Autodesk Inventor part; units mm, degrees
ref_plane "YZ Plane" through (0, 0, 0) normal (1, 0, 0) x (0, 1, 0)
ref_plane "XZ Plane" through (0, 0, 0) normal (0, 1, 0) x (-1, 0, 0)
ref_plane "XY Plane" through (0, 0, 0) normal (0, 0, 1) x (1, 0, 0)
sketch "Эскиз1" plane through (0, 0, 0) normal (1, 0, 0) x (0, 1, 0)
  line L0 (70.9825, 98.2222) -> (-59.0175, 98.2222)
  line L1 (-59.0175, 98.2222) -> (-59.0175, -105.7778)
  line L2 (-59.0175, -105.7778) -> (70.9825, -105.7778)
  line L3 (70.9825, -105.7778) -> (70.9825, 98.2222)
  circle A0 centre (-34.0175, 95.2222) radius 1.5
  circle A1 centre (-34.0175, -102.7778) radius 1.5
  circle A2 centre (12.9825, 95.2222) radius 1.5
  circle A3 centre (12.9825, -102.7778) radius 1.5
  circle A4 centre (32.9825, 95.2222) radius 1.5
  circle A5 centre (32.9825, -102.7778) radius 1.5
  line L4 (-59.0175, -105.7778) -> (70.9825, -105.7778)
  line L5 (70.9825, -105.7778) -> (70.9825, -127.7504)
  line L6 (70.9825, -127.7504) -> (-59.0175, -127.7504)
  line L7 (-59.0175, -127.7504) -> (-59.0175, -105.7778)
  point P0 (0, 0)
  dimension "d0" = 204
  dimension "d1" = 130
  dimension "d2" = 3
  dimension "d3" = 25
  dimension "d4" = 25
  dimension "d5" = 3
  dimension "d6" = 3
  dimension "d7" = 3
  dimension "d8" = 72
  dimension "d9" = 3
  dimension "d10" = 3
  dimension "d11" = 3
  dimension "d12" = 72
  dimension "d13" = 3
  dimension "d14" = 3
  dimension "d15" = 20
  dimension "d16" = 3
  dimension "d17" = 3
  dimension "d18" = 20
extrude "Выдавливание1" add sketch "Эскиз1" along normal blind 4
sketch "Эскиз2" plane through (0, 0, 0) normal (-1, 0, 0) x (0, 0, 1)
  circle A0 centre (-112.7504, -20.3037) radius 1.5
  circle A1 centre (25.0776, -20.3037) radius 1.5
  line L0 (98.2222, -59.0175) -> (-105.7778, -59.0175)
  circle A2 centre (-112.7504, 39.6963) radius 1.5
  circle A3 centre (25.0776, 39.6963) radius 1.5
  line L1 (98.2222, 70.9825) -> (98.2222, -59.0175)
  circle A4 centre (-102.7778, 12.9825) radius 1.5
  line L2 (-105.7778, -59.0175) -> (-105.7778, 70.9825)
  line L3 (-105.7778, 70.9825) -> (98.2222, 70.9825)
  line L4 (-127.7504, -59.0175) -> (-127.7504, 70.9825)
  circle A5 centre (-30.9224, 29.6963) radius 1.5
  point P0 (0, 0)
  point P1 (98.2222, 5.9825)
  dimension "d21" = 137.828
  dimension "d22" = 3
  dimension "d23" = 3
  dimension "d26" = 3
  dimension "d27" = 3
  dimension "d28" = 137.828
  dimension "d29" = 60
  dimension "d30" = 60
  dimension "d37" = 31.2861
  dimension "d38" = 31.2861
  dimension "d47" = 15
  dimension "d48" = 15
  dimension "d49" = 3
  dimension "d50" = 10
  dimension "d51" = 56
extrude "Выдавливание2" cut sketch "Эскиз2" against normal blind 5 contours A0 | A1 | A2 | A3 | A5
sketch "Эскиз3" plane through (0, 0, 0) normal (-1, 0, 0) x (0, 0, 1)
  line L0 (11.8903, 60.0049) -> (-3.1097, 60.0049) construction
  line L1 (11.8903, 67.5049) -> (-3.1097, 67.5049)
  line L2 (-3.1097, 52.5049) -> (11.8903, 52.5049)
  arc A0 (11.8903, 52.5049) -> (11.8903, 67.5049) centre (11.8903, 60.0049) ccw
  arc A1 (-3.1097, 67.5049) -> (-3.1097, 52.5049) centre (-3.1097, 60.0049) ccw
  line L3 (65.5667, 60.0049) -> (51.5667, 60.0049) construction
  line L4 (65.5667, 63.2549) -> (51.5667, 63.2549)
  line L5 (51.5667, 56.7549) -> (65.5667, 56.7549)
  arc A2 (65.5667, 56.7549) -> (65.5667, 63.2549) centre (65.5667, 60.0049) ccw
  arc A3 (51.5667, 63.2549) -> (51.5667, 56.7549) centre (51.5667, 60.0049) ccw
  line L6 (-50.6502, 60.0049) -> (-64.6502, 60.0049) construction
  line L7 (-50.6502, 63.2549) -> (-64.6502, 63.2549)
  line L8 (-64.6502, 56.7549) -> (-50.6502, 56.7549)
  arc A4 (-50.6502, 56.7549) -> (-50.6502, 63.2549) centre (-50.6502, 60.0049) ccw
  arc A5 (-64.6502, 63.2549) -> (-64.6502, 56.7549) centre (-64.6502, 60.0049) ccw
  line L9 (35.934, -50.5903) -> (-109.1416, -50.5903) construction
  line L10 (35.934, -47.1293) -> (-109.1416, -47.1293)
  line L11 (-109.1416, -54.0514) -> (35.934, -54.0514)
  arc A6 (35.934, -54.0514) -> (35.934, -47.1293) centre (35.934, -50.5903) ccw
  arc A7 (-109.1416, -47.1293) -> (-109.1416, -54.0514) centre (-109.1416, -50.5903) ccw
  point P0 (0, 0)
  point P1 (4.3903, 60.0049)
  point P2 (58.5667, 60.0049)
  point P3 (-57.6502, 60.0049)
  point P4 (-36.6038, -50.5903)
  dimension "d39" = 14
  dimension "d40" = 14
  dimension "d41" = 6.5
  dimension "d42" = 6.5
  dimension "d43" = 15
  dimension "d44" = 15
extrude "Выдавливание3" cut sketch "Эскиз3" against normal through all
sketch "Эскиз4" plane through (0, 0, 0) normal (-1, 0, 0) x (0, 0, 1)
  point P0 (0, 0)
sketch "Эскиз5" plane through (0, 0, 0) normal (-1, 0, 0) x (0, 0, 1)
  line L0 (-105.7778, -14.0175) -> (-99.7778, -14.0175)
  line L1 (-99.7778, -14.0175) -> (-99.7778, -29.0175)
  line L2 (-99.7778, -29.0175) -> (-105.7778, -29.0175)
  line L3 (-105.7778, -29.0175) -> (-105.7778, -14.0175)
  line L4 (-105.7778, 60.9825) -> (-99.7778, 60.9825)
  line L5 (-99.7778, 60.9825) -> (-99.7778, 45.9825)
  line L6 (-99.7778, 45.9825) -> (-105.7778, 45.9825)
  line L7 (-105.7778, 45.9825) -> (-105.7778, 60.9825)
  line L8 (92.2222, -14.0175) -> (98.2222, -14.0175)
  line L9 (98.2222, -14.0175) -> (98.2222, -29.0175)
  line L10 (98.2222, -29.0175) -> (92.2222, -29.0175)
  line L11 (92.2222, -29.0175) -> (92.2222, -14.0175)
  line L12 (92.2222, 60.9825) -> (98.2222, 60.9825)
  line L13 (98.2222, 60.9825) -> (98.2222, 45.9825)
  line L14 (98.2222, 45.9825) -> (92.2222, 45.9825)
  line L15 (92.2222, 45.9825) -> (92.2222, 60.9825)
  point P0 (0, 0)
extrude "Выдавливание4" cut sketch "Эскиз5" against normal through all
properties part number "крышка"
Check sheet for the modelled part. Datum: model origin and axes. Units: mm. A direction names the side the tool comes from. Coordinates: 2 decimals unless noted, no trailing zeros. Order: outer loops, then holes, each group sorted by start corner. A loop starts at its lowest first (then second) coordinate and runs counter-clockwise, first axis right, second up. Notation, with made-up numbers: (53.5, 45.5) -> (78.5, 45.5) arc R38 ccw to (78.5, 84.5) -> close; hole circle Ø3 at (11.5, 50.5). An arc over 180 degrees is marked (long way). Write each question's results on one line, items separated by ' | '. Start each with the question number.
1) Section check A-A (z = 3.5). Enter the section's corners in (x, y), and give its area (3 significant figures).
2) Draft check along Y on faces 1 (the face through (2, 53, 92.222)), 2 (the face through (2, 70.982, -16)), 3 (the face through (2, -44, 98.222)). Enter one of: pulls with the +Y half, pulls with the -Y half, needs draft (parallel to the pull), parting line crosses it, or undercut.
3) Section check B-B (y = 48.5). Enter the section's corners in (x, z).
4) Section check D-D (x = 2.65). Count the separate pieces of the cut face and the enclosed holes in it, and give its area (3 significant figures).
5) Set-up check for faces 4 (the face through (4, 5, -13)), 5 (the face through (2, -54.051, -38)), 6 (the face through (2, -14.018, 95)): record each of +Z, -Z, +X, -X, +Y, -Y from which the full face is reachable in a straight line by a thin tool's end or side.
6) Section check C-C (z = -90.5). Enter the section's corners in (x, y), and give its area (3 significant figures).
7) Material ranges on line 1 along Y through (x, z) = (2.55, -69); line 2 along Y through (x, z) = (1.15, 60); line 3 along Y through (x, z) = (0.35, -31), recorded low to high.
8) Depth check by flat-ended pin: pin 1 (5 mm diameter, centred on y = 32.98, z = -102.78, fed in from -X); pin 2 (1.8 mm diameter, centred on y = -34.02, z = -102.78, fed in from +X). Enter the tip coordinate at first touch or a pass-through.
Checked values:
1) outline: (0, -59.02) -> (4, -59.02) -> (4, -54.05) -> (0, -54.05) -> close; (0, -47.13) -> (4, -47.13) -> (4, 52.5) -> (0, 52.5) -> close; (0, 67.5) -> (4, 67.5) -> (4, 70.98) -> (0, 70.98) -> close | area: 432 mm²
2) face 1: undercut | face 2: pulls with the +Y half | face 3: needs draft
3) outline: (0, -127.75) -> (4, -127.75) -> (4, -105.78) -> (0, -105.78) -> close; (0, -99.78) -> (4, -99.78) -> (4, 92.22) -> (0, 92.22) -> close
4) separate pieces: 1 | enclosed holes: 17 | area: 27,200 mm²
5) face 4: +Z, -Z, +X, +Y, -Y | face 5: +X, -X | face 6: +Z, +X, -X
6) outline: (0, -59.02) -> (4, -59.02) -> (4, -54.05) -> (0, -54.05) -> close; (0, -47.13) -> (4, -47.13) -> (4, 70.98) -> (0, 70.98) -> close | area: 492 mm²
7) line 1: -59.02 to -54.05, -47.13 to 70.98 | line 2: -59.02 to 56.75, 63.25 to 70.98 | line 3: -59.02 to -54.05, -47.13 to 28.2, 31.19 to 70.98
8) pin 1: x = 0 | pin 2: through
